Can you work these out from the model? Positions are in its coordinate system, mm. Face numbers are marked on the shaded views. A direction names the side the tool comes from. Give positions to 0.01 mm unless a question says otherwise; leave off trailing zeros. Order: outer loops, then holes, each group sorted by start corner. A loop starts at its lowest first (then second) coordinate and runs counter-clockwise, first axis right, second up. Notation, with made-up numbers: M -8,28.25 L 44,28.25 A14 cw 44,53.25 Z; hole C -19.75,54.5 d6. An arc over 180 degrees is marked long. Write each question's results on one line, items separated by ' | '.
from build123d import *

# Parameters (mm, degrees)
SKETCH1_W                   = 70
SKETCH1_H                   = 80
BOSS_EXTRUDE1_DEPTH         = 1
SKETCH2_W                   = 45.5
SKETCH2_H                   = 48
BOSS_EXTRUDE2_DEPTH         = 13
LO_M3_BAT_DRIVER_DEPTH      = 55.717456081
LO_M3_BAT_DRIVER_DEPTH_BACK = 55.717456081
SKETCH3_R                   = 1.7


with BuildPart() as part:
    # Sketch1 → Boss-Extrude1 (new body)
    with BuildSketch(Plane.XY):
        Rectangle(SKETCH1_W, SKETCH1_H)
    extrude(amount=-BOSS_EXTRUDE1_DEPTH)

    # Sketch2 → Boss-Extrude2 (add)
    with BuildSketch(Plane.XY):
        Rectangle(SKETCH2_W, SKETCH2_H)
    extrude(amount=-BOSS_EXTRUDE2_DEPTH)

    # Sketch3 → Lo_M3_bat_driver (cut, two sides: drawn at the far end of the back side and taken through both)
    with BuildSketch(Plane.XY.offset(-LO_M3_BAT_DRIVER_DEPTH_BACK)):
        with Locations(Location((-15, -37, 0), (0, 0, 180))):
            Circle(SKETCH3_R)
        with Locations(Location((-15, 37, 0), (0, 0, 180))):
            Circle(SKETCH3_R)
        with Locations(Location((15, -37, 0), (0, 0, 180))):
            Circle(SKETCH3_R)
        with Locations(Location((15, 37, 0), (0, 0, 180))):
            Circle(SKETCH3_R)
    extrude(amount=LO_M3_BAT_DRIVER_DEPTH + LO_M3_BAT_DRIVER_DEPTH_BACK, mode=Mode.SUBTRACT)


solid = part.part
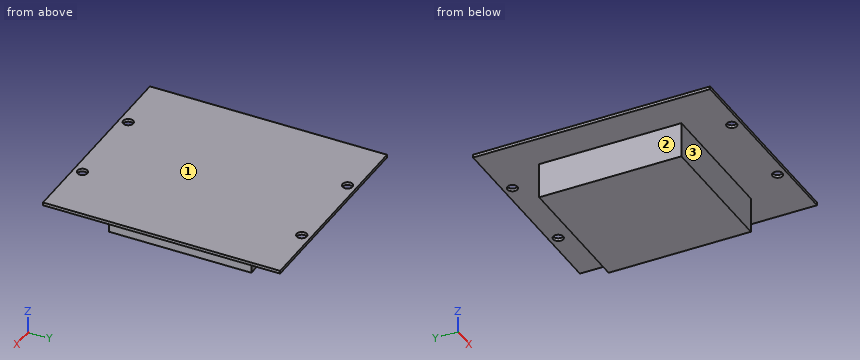
(1) Imagine slicing it at C-C, the plane x = 2. Write out the boundary of the cut face in (y, z), plus the area to 3 significant figures.
Data:
outline: M -40,-1 L -24,-1 L -24,-13 L 24,-13 L 24,-1 L 40,-1 L 40,0 L -40,0 Z | area: 656 mm2
(2) I need wall thicknesses on L1, parallel to Y at x = 15, z = -0.7; L2, parallel to Z at x = 21, y = 30; L3, parallel to X at y = 5, z = -7.75. Which ranges of each line are inside material? Lowest first, please. Write a range as from..to.
Data:
L1: y = -40..-38.7, -35.3..35.3, 38.7..40 | L2: z = -1..0 | L3: x = -22.75..22.75
(3) Imagine slicing it at A-A, the plane y = 37. Write out the boundary of the cut face in (x, z).
Data:
outline: M -35,-1 L -16.7,-1 L -16.7,0 L -35,0 Z; M -13.3,-1 L 13.3,-1 L 13.3,0 L -13.3,0 Z; M 16.7,-1 L 35,-1 L 35,0 L 16.7,0 Z
(4) Will these pins go through, and if not, where does the flat tip stop? P1, Ø1, axis at y = -20.5, z = -2, coming from the +X side; P2, Ø4, axis at x = 15, y = 37, coming from the -Z side; P3, Ø2, axis at y = -5.5, z = -11, coming from the -X side.
Data:
P1: stops at x = 22.75 | P2: stops at z = -1 | P3: stops at x = -22.75
(5) For the marked faces 1, 2 and 3, which set-ups out of +Z, -Z, +X, -X, +Y, -Y let a thin tool reach every point of the face, with its end or its side?
Data:
face 1: +Z, +X, -X, +Y, -Y | face 2: -Z, -X, +Y, -Y | face 3: -Z, +X, -X, -Y
(6) Imagine slicing it at B-B, the plane x = -15. Write out the boundary of the cut face in (y, z).
Data:
outline: M -40,-1 L -38.7,-1 L -38.7,0 L -40,0 Z; M -35.3,-1 L -24,-1 L -24,-13 L 24,-13 L 24,-1 L 35.3,-1 L 35.3,0 L -35.3,0 Z; M 38.7,-1 L 40,-1 L 40,0 L 38.7,0 Z
(7) Imagine slicing it at D-D, the plane y = 17.5. Write out the boundary of the cut face in (x, z).
Data:
outline: M -35,-1 L -22.75,-1 L -22.75,-13 L 22.75,-13 L 22.75,-1 L 35,-1 L 35,0 L -35,0 Z
